Can you work these out from the model? Positions are in its coordinate system, mm. A direction names the side the tool comes from. Give positions to 0.01 mm unless a question says otherwise; leave off trailing zeros. Loops run counter-clockwise (first coordinate to the right, second up) from the corner with the lowest first, then second, coordinate; pieces in that order, holes last. Notation, with made-up numbers: (-33, -29.75) - (22, -29.75) arc R9 ccw to (22, -20.75) - close; hole circle Ø7 at (68.5, -28.75). An arc over 180 degrees is marked (long way). Use a Markdown table: item, result. Add a question column.
```python
from build123d import *

# Parameters (mm, degrees)
SKETCH1_W                = 18
SKETCH1_H                = 10
SKETCH1_W_2              = 14
SKETCH1_H_2              = 6
BOSS_EXTRUDE1_DEPTH      = 6
BOSS_EXTRUDE2_DEPTH      = 34
SKETCH3_W                = 12
SKETCH3_H                = 10
SKETCH3_W_2              = 8
BOSS_EXTRUDE3_DEPTH      = 2
BOSS_EXTRUDE4_DEPTH      = 3
BOSS_EXTRUDE4_DEPTH_BACK = 3
CHAMFER1_SIZE            = 1
CHAMFER2_SIZE            = 1
SKETCH5_R                = 1.5
CUT_EXTRUDE1_DEPTH       = 48.116875958


with BuildPart() as part:
    # Sketch1 → Boss-Extrude1 (new body)
    with BuildSketch(Plane(origin=(0, 0, 0), x_dir=(1, 0, 0), z_dir=(0, 1, 0))):
        with Locations((9, 5)):
            Rectangle(SKETCH1_W, SKETCH1_H)
        with Locations((9, 5)):
            Rectangle(SKETCH1_W_2, SKETCH1_H_2, mode=Mode.SUBTRACT)
    extrude(amount=BOSS_EXTRUDE1_DEPTH)

    # Sketch2 → Boss-Extrude2 (add)
    with BuildSketch(Plane(origin=(0, 6, 0), x_dir=(1, 0, 0), z_dir=(0, 1, 0))):
        Polygon((0, 10), (0, 0), (8, 0), (8, 2), (2, 2), (2, 8), (8, 8), (8, 10), align=None)
    extrude(amount=BOSS_EXTRUDE2_DEPTH)

    # Sketch3 → Boss-Extrude3 (add)
    with BuildSketch(Plane(origin=(0, 0, 0), x_dir=(1, 0, 0), z_dir=(0, 1, 0))):
        with Locations((-6, 5)):
            Rectangle(SKETCH3_W, SKETCH3_H)
        with Locations((22, 5)):
            Rectangle(SKETCH3_W_2, SKETCH3_H)
    extrude(amount=BOSS_EXTRUDE3_DEPTH)

    # Sketch4 → Boss-Extrude4 (add, two sides: drawn at the far end of the back side and taken through both)
    with BuildSketch(Plane.XY.offset(-5).offset(-BOSS_EXTRUDE4_DEPTH_BACK)):
        Polygon((0, 2), (-4, 2), (0, 22), align=None)
    extrude(amount=BOSS_EXTRUDE4_DEPTH + BOSS_EXTRUDE4_DEPTH_BACK)

    # Chamfer1
    chamfer1_edges = [part.edges().sort_by_distance(p)[0] for p in [
        (8, 23, -10),
        (8, 23, 0),
        (-12, 1, -10),
        (-12, 1, 0),
        (26, 1, 0),
        (26, 1, -10),
        (0, 21, -10),
        (18, 4, -10),
        (18, 4, 0),
        (0, 21, 0),
    ]]
    chamfer(chamfer1_edges, length=CHAMFER1_SIZE)

    # Chamfer2
    chamfer2_edges = [part.edges().sort_by_distance(p)[0] for p in [
        (-2, 12, -8),
        (-2, 12, -2),
    ]]
    chamfer(chamfer2_edges, length=CHAMFER2_SIZE)

    # Sketch5 → Cut-Extrude1 (cut, through all)
    with BuildSketch(Plane(origin=(0, 2, 0), x_dir=(1, 0, 0), z_dir=(0, 1, 0))):
        with Locations(Location((-9, 5, 0), (0, 0, 270))):
            Circle(SKETCH5_R)
        with Locations(Location((23, 5, 0), (0, 0, 270))):
            Circle(SKETCH5_R)
    extrude(amount=-CUT_EXTRUDE1_DEPTH, mode=Mode.SUBTRACT)


solid = part.part
```
1. Suppose I cut it at D-D (x = 9). List the corners of the cut face in (y, z) for me, and give its area (3 significant figures).
2. Suppose I cut it at A-A (z = -5). List the corners of the cut face in (x, y) for me.
3. Will these pins go through, and if not, where does the flat tip stop? P1, Ø1.5, axis at x = -1, y = 6.5, coming from the +Z side; P2, Ø1.5, axis at y = 13.5, z = -3, coming from the -X side; P3, Ø1.5, axis at y = 28, z = -8, coming from the -X side; P4, Ø2, axis at x = 10, z = -4, coming from the +Y side.
4. If we mould it in two halves opening along X, with no side actions, what happens to faces 4 (the face through (17.5, 4, -9.5)), 5 (the face through (6.7, 0, -8.4)), 6 (the face through (24.487, 1.014, -5.195))? For each: released by +X, released by -X, zero draft, split by the parting line, or undercut.
5. Suppose I cut it at B-B (x = -9). List the corners of the cut face in (y, z) for me, and give its area (3 significant figures).
6. Please list where these lines run through material, in increasing order: line 1 along X through (y, z) = (0.5, -5); line 2 along Z through (x, y) = (4, 35.5); line 3 along X through (y, z) = (17, -5.5). Write a range as [from, to].
7. On a 3-axis mill with a long thin cutter (end or side, diameter ignored), from which of +Z, -Z, +X, -X, +Y, -Y can I reach the whole of each face in a straight line? I mean faces 1 (the face through (17.5, 4, -0.5)), 2 (the face through (6, 20, -8)), 3 (the face through (0.5, 21.3, -9.5)). Say none if no direction works.
8. Suppose I cut it at C-C (y = 25). List the corners of the cut face in (x, z) for me, and give its area (3 significant figures).
Results below:
| question | item | result |
|---|---|---|
| 1 | outline | (0, -10) - (6, -10) - (6, -8) - (0, -8) - close; (0, -2) - (6, -2) - (6, 0) - (0, 0) - close |
| 1 | area | 24.0 mm² |
| 2 | outline | (-12, 0) - (-10.5, 0) - (-10.5, 2) - (-12, 2) - close; (-7.5, 0) - (2, 0) - (2, 40) - (0, 40) - (0, 22) - (-4, 2) - (-7.5, 2) - close; (16, 0) - (21.5, 0) - (21.5, 2) - (18, 2) - (18, 6) - (16, 6) - close; (24.5, 0) - (26, 0) - (26, 2) - (24.5, 2) - close |
| 3 | P1 | z = -2 |
| 3 | P2 | x = -1.85 |
| 3 | P3 | x = 0 |
| 3 | P4 | through |
| 4 | face 4 | released by +X |
| 4 | face 5 | zero draft |
| 4 | face 6 | undercut |
| 5 | outline | (0, -10) - (2, -10) - (2, -6.5) - (0, -6.5) - close; (0, -3.5) - (2, -3.5) - (2, 0) - (0, 0) - close |
| 5 | area | 14.0 mm² |
| 6 | line 1 | [-12, -10.5], [-7.5, 2], [16, 21.5], [24.5, 26] |
| 6 | line 2 | [-10, -8], [-2, 0] |
| 6 | line 3 | [-1, 2] |
| 7 | face 1 | +Z, +X, +Y |
| 7 | face 2 | +Y, -Y |
| 7 | face 3 | -Z, -X, +Y |
| 8 | outline | (0, -9) - (1, -10) - (7, -10) - (8, -9) - (8, -8) - (2, -8) - (2, -2) - (8, -2) - (8, -1) - (7, 0) - (1, 0) - (0, -1) - close |
| 8 | area | 42.0 mm² |
